Design review of the part built by this model. Coordinates are the model's own, in mm. A direction names the side the tool comes from. Coordinates: 2 decimals unless noted, no trailing zeros. Loops run counter-clockwise (first coordinate to the right, second up) from the corner with the lowest first, then second, coordinate; pieces in that order, holes last. Notation, with made-up numbers: M 0.25,10 L 49.25,10 A21 cw 49.25,43 Z; hole C -21,78.25 d11. An arc over 180 degrees is marked long. Answer as a JSON object with one key per item and string values. Group by question number.
1. Consider section C-C (z = -29). State the section outline as (x, y) points, then the cut area to 4 significant figures.
2. Machinability: for faces 4 (the flat face through (-2, 93.75, -13)), 5 (the cylindrical face through (-94, 91, -18)), which of the approach directions +Z, -Z, +X, -X, +Y, -Y give a long, thin tool a straight path to every point of the face, cutting with its end or side? Answer none if there is none.
3. To check wall thickness, follow probe 1 along Z at (x, y) = (101, -91); probe 2 along Z at (x, y) = (17, -90.2); probe 3 along X at (y, z) = (-61, -4). State the ranges of each line that lie inside material, in increasing order.
4. Consider section A-A (x = 101). State the section outline as (y, z) points.
5. Consider section B-B (x = 63). State the section outline as (y, z) points, then the cut area to 3 significant figures.
6. Insertion check: pin 1 (1.5 mm diameter, centred on x = 87, y = -65.5, fed in from -Z); pin 2 (8.5 mm diameter, centred on y = -76.5, z = -4.5, fed in from -X); pin 3 (2.5 mm diameter, centred on x = 85, z = -1.5, fed in from +Y). Each pin has a flat end and moves straight along its axis. Give the tip position at first contact, or say it passes through.
7. Draft analysis for pull direction Z (two halves, no side actions). For faces 1 (the flat face through (-1, -88.75, -13)), 2 (the cylindrical face through (-94, -91, -18)), 3 (the flat face through (46, 0, -35)), state which applies: +Z half, -Z half, draft (parallel to the pull), parting line (faces both ways), or undercut.
8. Consider section D-D (y = 1). State the section outline as (x, z) points.
from build123d import *

# Parameters (mm, degrees)
F2_W      = 250
F2_H      = 250
F3_DEPTH  = 5
F4_W      = 5
F4_H      = 41.6666666667
F5_DEPTH  = 5
F6_W      = 250
F6_H      = 30
F7_DEPTH  = 5
F8_W      = 250
F8_H      = 30
F9_DEPTH  = 5
F11_R     = 2.5
F10_W     = 5
F10_H     = 187.5
F12_DEPTH = 35
F13_R     = 6
F13_R_2   = 7
F13_R_3   = 2.5
F14_DEPTH = 218.751
F15_R     = 2.6
F16_DEPTH = 40.001


with BuildPart() as f3:
    # F2 (on Top) → F3 (new body)
    with BuildSketch(Plane.XY):
        Rectangle(F2_W, F2_H)
    extrude(amount=F3_DEPTH)

    # F4 (on face) → F5 (join)
    with BuildSketch(Plane(origin=(0, 0, 0), x_dir=(1, 0, 0), z_dir=(0, 0, -1))):
        with Locations((-85.8333333333, 72.9166666667)):
            Rectangle(F4_W, F4_H)
        with Locations((85.8333333333, 72.9166666667)):
            Rectangle(F4_W, F4_H)
        with Locations((-85.8333333333, -72.9166666667)):
            Rectangle(F4_W, F4_H)
        with Locations((85.8333333333, -72.9166666667)):
            Rectangle(F4_W, F4_H)
    extrude(amount=F5_DEPTH)

    # F6 (on face) → F7 (join)
    with BuildSketch(Plane(origin=(0, 93.75, 0), x_dir=(-1, 0, 0), z_dir=(0, 1, 0))):
        with Locations((0, -20)):
            Rectangle(F6_W, F6_H)
    extrude(amount=-F7_DEPTH)

    # F8 (on face) → F9 (join)
    with BuildSketch(Plane.XZ.offset(93.75)):
        with Locations((0, -20)):
            Rectangle(F8_W, F8_H)
    extrude(amount=-F9_DEPTH)

    # F11
    f11_edges = [f3.edges().sort_by_distance(p)[0] for p in [
        (85.833333, -88.75, -5),
        (-85.833333, -88.75, -5),
        (85.833333, 88.75, -5),
        (-85.833333, 88.75, -5),
    ]]
    fillet(f11_edges, radius=F11_R)

    # F10 (on face) → F12 (join, through all)
    with BuildSketch(Plane(origin=(0, 0, 0), x_dir=(1, 0, 0), z_dir=(0, 0, -1))):
        with Locations((44.1666666667, 0)):
            Rectangle(F10_W, F10_H)
        with Locations((-44.1666666667, 0)):
            Rectangle(F10_W, F10_H)
    extrude(amount=F12_DEPTH)

    # F13 (on face) → F14 (cut, through all)
    with BuildSketch(Plane(origin=(0, 93.75, 0), x_dir=(-1, 0, 0), z_dir=(0, 1, 0))):
        with Locations((0, -20)):
            Circle(F13_R)
        with Locations((-101, -18)):
            Circle(F13_R_2)
        with Locations((101, -18)):
            Circle(F13_R_2)
        with Locations((17, -20)):
            Circle(F13_R_3)
        with Locations((-17, -20)):
            Circle(F13_R_3)
    extrude(amount=-F14_DEPTH, mode=Mode.SUBTRACT)

    # F15 (on face) → F16 (cut, through all)
    with BuildSketch(Plane.XY.offset(5)):
        with Locations((-85, -21.333)):
            Circle(F15_R)
        with Locations((-115, 18.667)):
            Circle(F15_R)
        with Locations((115, -21.333)):
            Circle(F15_R)
        with Locations((85, 18.667)):
            Circle(F15_R)
    extrude(amount=-F16_DEPTH, mode=Mode.SUBTRACT)


solid = f3.part
Findings below:
{
 "1": {"outline": "M -125,-93.75 L 125,-93.75 L 125,-88.75 L 46.67,-88.75 L 46.67,88.75 L 125,88.75 L 125,93.75 L -125,93.75 L -125,88.75 L -46.67,88.75 L -46.67,-88.75 L -125,-88.75 Z; hole M -41.67,-88.75 L 41.67,-88.75 L 41.67,88.75 L -41.67,88.75 Z", "area": "4,275 mm^2"},
 "2": {"face 4": "-Z, +X, -X, +Y", "face 5": "+Y, -Y"},
 "3": {"probe 1": "z = -35 to -25, -11 to -5, 0 to 5", "probe 2": "z = -35 to -22.5, -17.5 to -5, 0 to 5", "probe 3": "x = -88.33 to -83.33, -46.67 to -41.67, 41.67 to 46.67, 83.33 to 88.33"},
 "4": {"outline": "M -125,0 L 125,0 L 125,5 L -125,5 Z; M -93.75,-35 L -88.75,-35 L -88.75,-25 L -93.75,-25 Z; M -93.75,-11 L -88.75,-11 L -88.75,-5 L -93.75,-5 Z; M 88.75,-35 L 93.75,-35 L 93.75,-25 L 88.75,-25 Z; M 88.75,-11 L 93.75,-11 L 93.75,-5 L 88.75,-5 Z"},
 "5": {"outline": "M -125,0 L 125,0 L 125,5 L -125,5 Z; M -93.75,-35 L -88.75,-35 L -88.75,-5 L -93.75,-5 Z; M 88.75,-35 L 93.75,-35 L 93.75,-5 L 88.75,-5 Z", "area": "1,550 mm^2"},
 "6": {"pin 1": "stops at z = -5", "pin 2": "stops at x = -88.33", "pin 3": "stops at y = 93.75"},
 "7": {"face 1": "draft", "face 2": "undercut", "face 3": "-Z half"},
 "8": {"outline": "M -125,0 L -46.67,0 L -46.67,-35 L -41.67,-35 L -41.67,0 L 41.67,0 L 41.67,-35 L 46.67,-35 L 46.67,0 L 125,0 L 125,5 L -125,5 Z"}
}
